For this review, take the finished solid that the model builds, in its own axes (mm). A direction names the side the tool comes from. Coordinates: 2 decimals unless noted, no trailing zeros. Loops run counter-clockwise (first coordinate to the right, second up) from the corner with the lowest first, then second, coordinate; pieces in that order, holes last. Notation, with made-up numbers: (25, 8) -> (55, 8) arc R26 cw to (55, 47) -> close; hole circle Ø10 at (10, 30). An arc over 180 degrees is marked (long way). Use a Markdown table: item, result.
from build123d import *

# Parameters (mm, degrees)
F0_W     = 12
F0_H     = 5
F0_R     = 1.5
F0_H_2   = 30
F1_DEPTH = 2
F2_DEPTH = 6
F3_DEPTH = 20
F4_R     = 3
F5_DEPTH = 8.5
F4_R_2   = 5.75
F6_DEPTH = 5


with BuildPart() as f1:
    # F0 (on Top) → F1 (new body)
    with BuildSketch(Plane.XY):
        with Locations((6, 37.5)):
            Rectangle(F0_W, F0_H)
        with Locations((6, 38)):
            Circle(F0_R, mode=Mode.SUBTRACT)
        with Locations((6, 20)):
            Rectangle(F0_W, F0_H_2)
        with Locations((6, 2.5)):
            Rectangle(F0_W, F0_H)
        with Locations((6, 2)):
            Circle(F0_R, mode=Mode.SUBTRACT)
    extrude(amount=F1_DEPTH)

    # F0 (on Top) → F2 (join)
    with BuildSketch(Plane.XY):
        with Locations((6, 20)):
            Rectangle(F0_W, F0_H_2)
    extrude(amount=F2_DEPTH)

    # F0 (on Top) → F3 (join)
    with BuildSketch(Plane.XY):
        with Locations((6, 20)):
            Rectangle(F0_W, F0_H_2)
    extrude(amount=-F3_DEPTH)

    # F4 (on face) → F5 (join)
    with BuildSketch(Plane.XY.offset(6)):
        with Locations((6, 25)):
            Circle(F4_R)
    extrude(amount=F5_DEPTH)

    # F4 (on face) → F6 (join)
    with BuildSketch(Plane.XY.offset(6)):
        with Locations((6, 25)):
            Circle(F4_R_2)
        with Locations((6, 25)):
            Circle(F4_R, mode=Mode.SUBTRACT)
    extrude(amount=F6_DEPTH)


solid = f1.part
(1) For line 1 along Y through (x, z) = (6, 1.1); line 2 along Z through (x, y) = (1, 12.5); line 3 along Z through (x, y) = (4.5, 37), list the stretches that pass through material, from the lowest coordinate up.
Found:
| item | result |
|---|---|
| line 1 | y = 0 to 0.5, 3.5 to 36.5, 39.5 to 40 |
| line 2 | z = -20 to 6 |
| line 3 | z = 0 to 2 |
(2) Take a section at B-B on x = 5.5. Write out the cut boundary in (y, z), plus the area to 3 significant figures.
Found:
| item | result |
|---|---|
| outline | (0, 0) -> (0.59, 0) -> (0.59, 2) -> (0, 2) -> close; (3.41, 0) -> (5, 0) -> (5, -20) -> (35, -20) -> (35, 0) -> (36.59, 0) -> (36.59, 2) -> (35, 2) -> (35, 6) -> (30.73, 6) -> (30.73, 11) -> (27.96, 11) -> (27.96, 14.5) -> (22.04, 14.5) -> (22.04, 11) -> (19.27, 11) -> (19.27, 6) -> (5, 6) -> (5, 2) -> (3.41, 2) -> close; (39.41, 0) -> (40, 0) -> (40, 2) -> (39.41, 2) -> close |
| area | 867 mm^2 |
(3) For faces 5 (the face through (8.5, 22.5, 11)), 6 (the face through (6, 4, 2)), 7 (the face through (6, 5, -10)), list the 3-axis set-ups (+Z, -Z, +X, -X, +Y, -Y) from which the entire face can be reached by the end or side of a thin tool; tool diameter is ignored.
Found:
| item | result |
|---|---|
| face 5 | +Z |
| face 6 | +Z, +X, -X, -Y |
| face 7 | -Z, +X, -X, -Y |
(4) For pin 1 Ø1.2 at (x, z) = (5, 5) entering from +Y; pin 2 Ø1.5 at (x, y) = (7.5, 1.5) entering from +Z; pin 3 Ø2 at (x, z) = (8.5, 3.5) entering from -Y, all flat-tipped, find the tip position at first contact; note any pin that passes through.
Found:
| item | result |
|---|---|
| pin 1 | stops at y = 35 |
| pin 2 | stops at z = 2 |
| pin 3 | stops at y = 5 |
(5) Take a section at A-A on y = 38. Write out the cut boundary in (x, z).
Found:
| item | result |
|---|---|
| outline | (0, 0) -> (4.5, 0) -> (4.5, 2) -> (0, 2) -> close; (7.5, 0) -> (12, 0) -> (12, 2) -> (7.5, 2) -> close |
(6) Mouldability with a two-part tool opening along Y and no side actions: class faces 1 (the face through (4.8, 1.1, 1)), 2 (the face through (6, 5, 4)), 3 (the face through (6, 40, 1)), 4 (the face through (6, 36, 2)) as pulls with the +Y half, pulls with the -Y half, needs draft (parallel to the pull), parting line crosses it, or undercut.
Found:
| item | result |
|---|---|
| face 1 | undercut |
| face 2 | pulls with the -Y half |
| face 3 | pulls with the +Y half |
| face 4 | needs draft |
(7) Take a section at D-D on x = 2.5. Write out the cut boundary in (y, z).
Found:
| item | result |
|---|---|
| outline | (0, 0) -> (5, 0) -> (5, -20) -> (35, -20) -> (35, 0) -> (40, 0) -> (40, 2) -> (35, 2) -> (35, 6) -> (29.56, 6) -> (29.56, 11) -> (20.44, 11) -> (20.44, 6) -> (5, 6) -> (5, 2) -> (0, 2) -> close |
(8) Take a section at C-C on y = 25. Write out the cut boundary in (x, z).
Found:
| item | result |
|---|---|
| outline | (0, -20) -> (12, -20) -> (12, 6) -> (11.75, 6) -> (11.75, 11) -> (9, 11) -> (9, 14.5) -> (3, 14.5) -> (3, 11) -> (0.25, 11) -> (0.25, 6) -> (0, 6) -> close |
